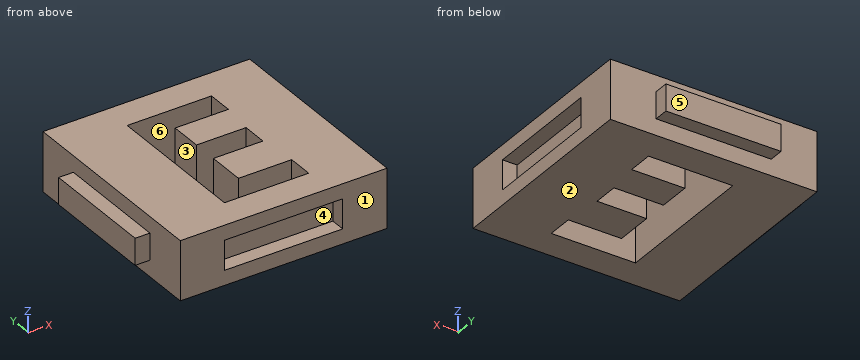
```python
from build123d import *

# Parameters (mm, degrees)
F0_W     = 35.56
F0_H     = 35.56
F1_DEPTH = 5.08
F2_W     = 19.812
F2_H     = 4.572
F3_DEPTH = 2.54
F4_W     = 19.812
F4_H     = 4.572
F5_DEPTH = 2.54
F6_W     = 20.32
F6_H     = 5.08
F7_DEPTH = 2.54
F8_W     = 20.32
F8_H     = 5.08
F9_DEPTH = 2.54


with BuildPart() as f1:
    # F0 (on Top) → F1 (new body, symmetric)
    with BuildSketch(Plane.XY):
        Rectangle(F0_W, F0_H)
        Polygon((7.6922092014, -8.2902777778), (7.6922092014, -12.7), (-6.8102647569, -12.7), (-6.8102647569, 12.4850260417), (7.6922092014, 12.4850260417), (7.6922092014, 8.1083767361), (-1.4689887153, 8.1083767361), (-1.4689887153, 2.5796875), (7.0583116319, 2.5796875), (7.0583116319, -1.7969618056), (-1.4689887153, -1.7969618056), (-1.4689887153, -8.2902777778), align=None, mode=Mode.SUBTRACT)
    extrude(amount=F1_DEPTH, both=True)

    # F2 (on face) → F3 (join)
    with BuildSketch(Plane(origin=(0, 17.78, 0), x_dir=(-1, 0, 0), z_dir=(0, 1, 0))):
        Rectangle(F2_W, F2_H)
    extrude(amount=F3_DEPTH)

    # F4 (on face) → F5 (join)
    with BuildSketch(Plane(origin=(-17.78, 0, 0), x_dir=(0, -1, 0), z_dir=(-1, 0, 0))):
        Rectangle(F4_W, F4_H)
    extrude(amount=F5_DEPTH)

    # F6 (on face) → F7 (cut)
    with BuildSketch(Plane.XZ.offset(17.78)):
        Rectangle(F6_W, F6_H)
    extrude(amount=-F7_DEPTH, mode=Mode.SUBTRACT)

    # F8 (on face) → F9 (cut)
    with BuildSketch(Plane.YZ.offset(17.78)):
        Rectangle(F8_W, F8_H)
    extrude(amount=-F9_DEPTH, mode=Mode.SUBTRACT)


solid = f1.part
```
Geometry check sheet. Reference: the model listing, model coordinates, mm. Face numbers are marked on the shaded views. A direction names the side the tool comes from. Give positions to 0.01 mm unless a question says otherwise; leave off trailing zeros. Order: outer loops, then holes, each group sorted by start corner. A loop starts at its lowest first (then second) coordinate and runs counter-clockwise, first axis right, second up. Notation, with made-up numbers: (8.25, -6) - (62.25, -6) arc R5 ccw to (62.25, -1) - close; hole circle Ø9 at (27, 44). An arc over 180 degrees is marked (long way). Answer in a Markdown table with one row per item. Add a question column.
Q1. Mould release check, pull along Y, two halves, no side actions. Record for the marked faces 1, 2 and 3: pulls with the +Y half, pulls with the -Y half, needs draft (parallel to the pull), parting line crosses it, or undercut.
Q2. Material ranges on probe 1 along Y at (x, z) = (5, 0); probe 2 along X at (y, z) = (-12.5, -1.75); probe 3 along Y at (x, z) = (1.5, -4.25), recorded low to high. Write a range as from..to.
Q3. Cross-section at A-A, the plane x = -5. Enter the section's corners in (y, z), then the cut area to 3 significant figures.
Q4. Cross-section at B-B, the plane y = -5. Enter the section's corners in (x, z), then the cut area to 3 significant figures.
Q5. Tool access check on the marked faces 4, 5 and 6. Record the directions out of +Z, -Z, +X, -X, +Y, -Y that give a thin tool (end or side, any length) a straight path to the whole face; none if there is none.
Q6. Gauge pin test, flat ends, axial feed: pin 1 (1 mm diameter, centred on y = -13.5, z = -0.5, fed in from -X); pin 2 (0.8 mm diameter, centred on x = -19, y = 2, fed in from -Z); pin 3 (2 mm diameter, centred on x = -19, z = 0.5, fed in from -Y). Record the tip position at first contact, or that the pin passes through.
Q7. Cross-section at D-D, the plane y = 12. Enter the section's corners in (x, z), then the cut area to 3 significant figures.
Q8. Cross-section at C-C, the plane z = 3.75. Enter the section's corners in (x, y).
Check values:
| question | item | result |
|---|---|---|
| 1 | face 1 | pulls with the -Y half |
| 1 | face 2 | needs draft |
| 1 | face 3 | undercut |
| 2 | probe 1 | y = -15.24..-12.7, -8.29..-1.8, 2.58..8.11, 12.49..20.32 |
| 2 | probe 2 | x = -17.78..-6.81, 7.69..17.78 |
| 2 | probe 3 | y = -17.78..-12.7, -8.29..-1.8, 2.58..8.11, 12.49..17.78 |
| 3 | outline | (-17.78, -5.08) - (-12.7, -5.08) - (-12.7, 5.08) - (-17.78, 5.08) - (-17.78, 2.54) - (-15.24, 2.54) - (-15.24, -2.54) - (-17.78, -2.54) - close; (12.49, -5.08) - (17.78, -5.08) - (17.78, -2.29) - (20.32, -2.29) - (20.32, 2.29) - (17.78, 2.29) - (17.78, 5.08) - (12.49, 5.08) - close |
| 3 | area | 104 mm^2 |
| 4 | outline | (-20.32, -2.29) - (-17.78, -2.29) - (-17.78, -5.08) - (-6.81, -5.08) - (-6.81, 5.08) - (-17.78, 5.08) - (-17.78, 2.29) - (-20.32, 2.29) - close; (-1.47, -5.08) - (17.78, -5.08) - (17.78, -2.54) - (15.24, -2.54) - (15.24, 2.54) - (17.78, 2.54) - (17.78, 5.08) - (-1.47, 5.08) - close |
| 4 | area | 306 mm^2 |
| 5 | face 4 | -Y |
| 5 | face 5 | +Z, -Z, +X, -X, +Y |
| 5 | face 6 | +Z, -Z |
| 6 | pin 1 | stops at x = -17.78 |
| 6 | pin 2 | stops at z = -2.29 |
| 6 | pin 3 | stops at y = -9.91 |
| 7 | outline | (-17.78, -5.08) - (-6.81, -5.08) - (-6.81, 5.08) - (-17.78, 5.08) - close; (7.69, -5.08) - (17.78, -5.08) - (17.78, 5.08) - (7.69, 5.08) - close |
| 7 | area | 214 mm^2 |
| 8 | outline | (-17.78, -17.78) - (17.78, -17.78) - (17.78, 17.78) - (-17.78, 17.78) - close; hole (-6.81, -12.7) - (7.69, -12.7) - (7.69, -8.29) - (-1.47, -8.29) - (-1.47, -1.8) - (7.06, -1.8) - (7.06, 2.58) - (-1.47, 2.58) - (-1.47, 8.11) - (7.69, 8.11) - (7.69, 12.49) - (-6.81, 12.49) - close |
